Check sheet for the modelled part. Datum: model origin and axes. Units: mm. A direction names the side the tool comes from. Round coordinates to 2 decimals unless told otherwise and drop trailing zeros. Order: outer loops, then holes, each group sorted by start corner. A loop starts at its lowest first (then second) coordinate and runs counter-clockwise, first axis right, second up. Notation, with made-up numbers: (24.5, -1.75) -> (41.5, -1.75) arc R27 cw to (41.5, 19.25) -> close; hole circle Ø7 at (66, -34.5). An arc over 180 degrees is marked (long way). Answer in a Markdown table with one row per item. Add a question column.
1. Sectioned sample at B-B, the plane z = 17. Record the boundary of the cut face in (x, y).
2. Access from +Z, -Z, +X, -X, +Y, -Y to the whole of each face (thin tool, end or side, straight path). Record for faces 1 (the cylindrical face through (42.43, -4.93, -58.73)), 2 (the cylindrical face through (0.46, -7.05, 62.7)).
3. Sectioned sample at A-A, the plane x = -42. Record the boundary of the cut face in (y, z), then the cut area to 3 significant figures.
4. Draft check along Z on faces 3 (the flat face through (-1, -5, -70)), 4 (the conical face through (0.2, -4.69, 54.56)), 5 (the flat face through (-50, -5, -1)), 6 (the cylindrical face through (28.226, -4.93, 52.783)). Enter one of: +Z half, -Z half, draft (parallel to the pull), parting line (faces both ways), or undercut.
5. Depth check by flat-ended pin: P1, Ø5, axis at x = 0, y = -5, coming from the +Z side; P2, Ø6, axis at x = -42, z = -62, coming from the +Y side. Enter the tip coordinate at first touch or a pass-through.
6. Material ranges on L1, parallel to Z at x = 30, y = -2.75; L2, parallel to Z at x = 42, y = -6; L3, parallel to Z at x = -25, y = -4.5, recorded low to high. Write a range as from..to.
```python
from build123d import *

# Parameters (mm, degrees)
F0_W     = 100
F0_H     = 140
F0_R     = 11
F1_DEPTH = 10
F4_D     = 4.2
F4_DEPTH = 14.4
F4_TIP   = 1.2618073
F5_D     = 6.6


with BuildPart() as f1:
    # F0 (on Front) → F1 (new body)
    with BuildSketch(Plane.XZ):
        Rectangle(F0_W, F0_H)
        with Locations((-25, 17)):
            Circle(F0_R, mode=Mode.SUBTRACT)
    extrude(amount=F1_DEPTH)

    # F4
    with Locations(Plane.XY.offset(70)):
        with Locations((0, -5)):
            Hole(F4_D / 2, depth=F4_DEPTH)
            with Locations((0, 0, -(F4_DEPTH + F4_TIP / 2))):  # 118° drill point
                Cone(0, F4_D / 2, F4_TIP, mode=Mode.SUBTRACT)

    # F5 (through all)
    with Locations(Plane.XZ.offset(10)):
        with Locations((30, 50), (30, 0), (-42, -62), (42, -62)):
            Hole(F5_D / 2)


solid = f1.part
```
Answer key:
| question | item | result |
|---|---|---|
| 1 | outline | (-50, -10) -> (-36, -10) -> (-36, 0) -> (-50, 0) -> close; (-14, -10) -> (50, -10) -> (50, 0) -> (-14, 0) -> close |
| 2 | face 1 | +Y, -Y |
| 2 | face 2 | +Z |
| 3 | outline | (-10, -70) -> (0, -70) -> (0, -65.3) -> (-10, -65.3) -> close; (-10, -58.7) -> (0, -58.7) -> (0, 70) -> (-10, 70) -> close |
| 3 | area | 1,330 mm² |
| 4 | face 3 | -Z half |
| 4 | face 4 | +Z half |
| 4 | face 5 | draft |
| 4 | face 6 | undercut |
| 5 | P1 | stops at z = 70 |
| 5 | P2 | passes through |
| 6 | L1 | z = -70..-3.3, 3.3..46.7, 53.3..70 |
| 6 | L2 | z = -70..-65.3, -58.7..70 |
| 6 | L3 | z = -70..6, 28..70 |
